```python
from build123d import *

# Parameters (mm, degrees)
F0_R     = 7.344689
F1_DEPTH = 15
F2_SIZE  = 5
F3_R     = 0.805214
F3_R_2   = 0.724696
F3_R_3   = 0.64417
F3_R_4   = 0.586207
F4_DEPTH = 25
F5_R     = 1.214251
F6_DEPTH = 25


with BuildPart() as f1:
    # F0 (on Top) → F1 (new body)
    with BuildSketch(Plane.XY):
        with Locations((-43.481596, 43.64264)):
            Circle(F0_R)
    extrude(amount=F1_DEPTH)

    # F2
    f2_edges = [f1.edges().sort_by_distance(p)[0] for p in [
        (-50.826285, 43.64264, 15),
    ]]
    chamfer(f2_edges, length=F2_SIZE)

    # F3 (on Top) → F4 (cut)
    with BuildSketch(Plane.XY):
        with Locations((-43.562695, 48.90348)):
            Circle(F3_R)
        with Locations((-43.562695, 38.838297)):
            Circle(F3_R_2)
        with Locations((-38.892448, 43.669585)):
            Circle(F3_R_3)
        with Locations((-48.555028, 43.669585)):
            Circle(F3_R_4)
    extrude(amount=F4_DEPTH, mode=Mode.SUBTRACT)

    # F5 (on Top) → F6 (cut)
    with BuildSketch(Plane.XY):
        with Locations((-43.492485, 43.788202)):
            Circle(F5_R)
    extrude(amount=F6_DEPTH, mode=Mode.SUBTRACT)


solid = f1.part
```
Check sheet for the modelled part. Datum: model origin and axes. Units: mm. Coordinates: 2 decimals unless noted, no trailing zeros. Write each loop counter-clockwise with the first axis right and the second up, starting at its lowest first coordinate (ties: lowest second). Pieces come first, ordered by that corner, then holes. Notation, with made-up numbers: (24.5, 29.25) - (46.5, 29.25) arc R9 ccw to (46.5, 39.25) - close; hole circle Ø1 at (66, 34). An arc over 180 degrees is marked (long way). One line per question, with ' | ' between items.
Item 1: Mould release check, pull along Y, two halves, no side actions. Record for faces 1 (the face through (-47.996, 43.846, 6.339)), 2 (the face through (-45.07, 36.47, 4.93)), 3 (the face through (-44.387, 44.609, 7.395)), 4 (the face through (-45, 43, 15)): pulls with the +Y half, pulls with the -Y half, needs draft (parallel to the pull), parting line crosses it, or undercut.
Determined:
face 1: undercut | face 2: parting line crosses it | face 3: undercut | face 4: needs draft
Item 2: Gauge pin test, flat ends, axial feed: P1, Ø1, axis at y = 40, z = 3, coming from the +X side; P2, Ø1.5, axis at x = -38.89, y = 43.67, coming from the +Z side; P3, Ø1, axis at x = -43.56, y = 48.9, coming from the -Z side; P4, Ø1, axis at x = -39, y = 46, coming from the +Z side. Record the tip position at first contact, or that the pin passes through.
Determined:
P1: stops at x = -36.84 | P2: stops at z = 13.5 | P3: passes through | P4: stops at z = 12.78
Item 3: Thickness scan on line 1 (Y direction, x = -43.5, z = 7.25); line 2 (Y direction, x = -43, z = 8.75); line 3 (Y direction, x = -42.5, z = 8.25). Record the ranges inside material, lowest first. Write a range as [from, to].
Determined:
line 1: y = [36.3, 38.12], [39.56, 42.57], [45, 48.1], [49.71, 50.99] | line 2: y = [36.31, 38.38], [39.29, 42.68], [44.9, 48.33], [49.48, 50.97] | line 3: y = [36.36, 43.09], [44.49, 50.92]
Item 4: Sectioned sample at A-A on z = 3.5. Record the boundary of the cut face in (x, y), plus the area to 3 significant figures.
Determined:
outline: circle Ø14.69 at (-43.48, 43.64); hole circle Ø1.17 at (-48.56, 43.67); hole circle Ø2.43 at (-43.49, 43.79); hole circle Ø1.61 at (-43.56, 48.9); hole circle Ø1.45 at (-43.56, 38.84); hole circle Ø1.29 at (-38.89, 43.67) | area: 159 mm2
